Input: part model. Units: mm. Frame: model coordinates. Face numbers are marked on the shaded views. A direction names the side the tool comes from. Round coordinates to 2 decimals unless told otherwise and drop trailing zeros. Order: outer loops, then holes, each group sorted by start corner. A loop starts at its lowest first (then second) coordinate and runs counter-clockwise, first axis right, second up. Notation, with made-up numbers: (-10.5, 30.5) - (-4.5, 30.5) arc R25 cw to (-4.5, 65.5) - close; hole circle Ø1 at (57.25, -8). An arc over 180 degrees is marked (long way). One line per item, written item: value. Start each with the question number.
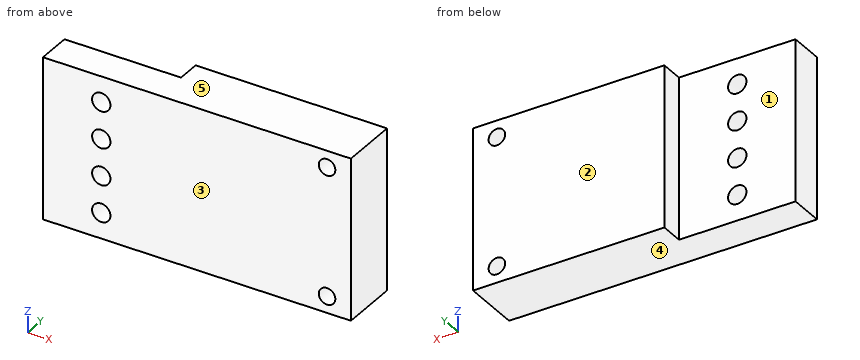
from build123d import *

# Parameters (mm, degrees)
F0_W     = 167.801
F0_H     = 88
F0_R     = 5
F0_R_2   = 4.5
F1_DEPTH = 31.375
F2_W     = 63.5
F2_H     = 12.7
F3_DEPTH = 88.001


with BuildPart() as f1:
    # F0 (on Front) → F1 (new body)
    with BuildSketch(Plane.XZ):
        with Locations((-1.279364, -11.298474)):
            Rectangle(F0_W, F0_H)
        with Locations((-53.429864, -41.298474)):
            Circle(F0_R, mode=Mode.SUBTRACT)
        with Locations((-53.429864, -21.298474)):
            Circle(F0_R, mode=Mode.SUBTRACT)
        with Locations((69.621136, -46.298474)):
            Circle(F0_R_2, mode=Mode.SUBTRACT)
        with Locations((-53.429864, -1.298474)):
            Circle(F0_R, mode=Mode.SUBTRACT)
        with Locations((-53.429864, 18.701526)):
            Circle(F0_R, mode=Mode.SUBTRACT)
        with Locations((69.621136, 23.701526)):
            Circle(F0_R_2, mode=Mode.SUBTRACT)
    extrude(amount=F1_DEPTH)

    # F2 (on face) → F3 (cut, through all)
    with BuildSketch(Plane(origin=(0, 0, -55.298474), x_dir=(1, 0, 0), z_dir=(0, 0, -1))):
        with Locations((-53.429864, 6.35)):
            Rectangle(F2_W, F2_H)
    extrude(amount=-F3_DEPTH, mode=Mode.SUBTRACT)


solid = f1.part
Item 1: Section query B-B on z = -10.5. Return loops of the section in (x, y) (3 decimals), and give its area (3 significant figures).
Item 2: Reachability of the marked faces 1 and 2 from +Z, -Z, +X, -X, +Y, -Y: full face, straight path, thin tool, end or side. Return the list, or none.
Item 3: First-contact query: pin 1 Ø6.5 at (y, z) = (-6, 4.5) entering from -X; pin 2 Ø13 at (x, z) = (-53.43, 18.7) entering from +Y; pin 3 Ø9 at (x, z) = (-53.43, -41.3) entering from +Y. Flat tips, straight axial feed; report the tip coordinate or a pass-through.
Item 4: Pull-direction query (Z, two-part tool) for the marked faces 3, 4 and 5; classes: released by +Z, released by -Z, zero draft, split by the parting line, or undercut.
Item 5: Section query D-D on x = -33. Return loops of the section in (y, z) (3 decimals).
Item 6: Section query A-A on y = -11. Return loops of the section in (x, z), and give its area (3 significant figures).
Item 7: Section query C-C on y = -27. Return loops of the section in (x, z).
Item 8: Line query: L1, parallel to Z at x = 73, y = -17; L2, parallel to X at y = -8, z = 2; L3, parallel to Y at x = -60.5, z = -18 (3 decimals). Output: solid intervals per line, ascending.
Geometry results:
1. outline: (-85.18, -31.375) - (82.621, -31.375) - (82.621, 0) - (-21.68, 0) - (-21.68, -12.7) - (-85.18, -12.7) - close
1. area: 4,460 mm^2
2. face 1: +Z, -Z, -X, +Y
2. face 2: +Z, -Z, +X, -X, +Y
3. pin 1: stops at x = -21.68
3. pin 2: stops at y = -12.7
3. pin 3: passes through
4. face 3: zero draft
4. face 4: released by -Z
4. face 5: released by +Z
5. outline: (-31.375, -55.298) - (-12.7, -55.298) - (-12.7, 32.702) - (-31.375, 32.702) - close
6. outline: (-21.68, -55.3) - (82.62, -55.3) - (82.62, 32.7) - (-21.68, 32.7) - close; hole circle Ø9 at (69.62, -46.3); hole circle Ø9 at (69.62, 23.7)
6. area: 9,050 mm^2
7. outline: (-85.18, -55.3) - (82.62, -55.3) - (82.62, 32.7) - (-85.18, 32.7) - close; hole circle Ø10 at (-53.43, -41.3); hole circle Ø10 at (-53.43, -21.3); hole circle Ø10 at (-53.43, -1.3); hole circle Ø10 at (-53.43, 18.7); hole circle Ø9 at (69.62, -46.3); hole circle Ø9 at (69.62, 23.7)
8. L1: z = -55.3 to -49.27, -43.33 to 20.73, 26.67 to 32.7
8. L2: x = -21.68 to 82.62
8. L3: y = -31.375 to -12.7
